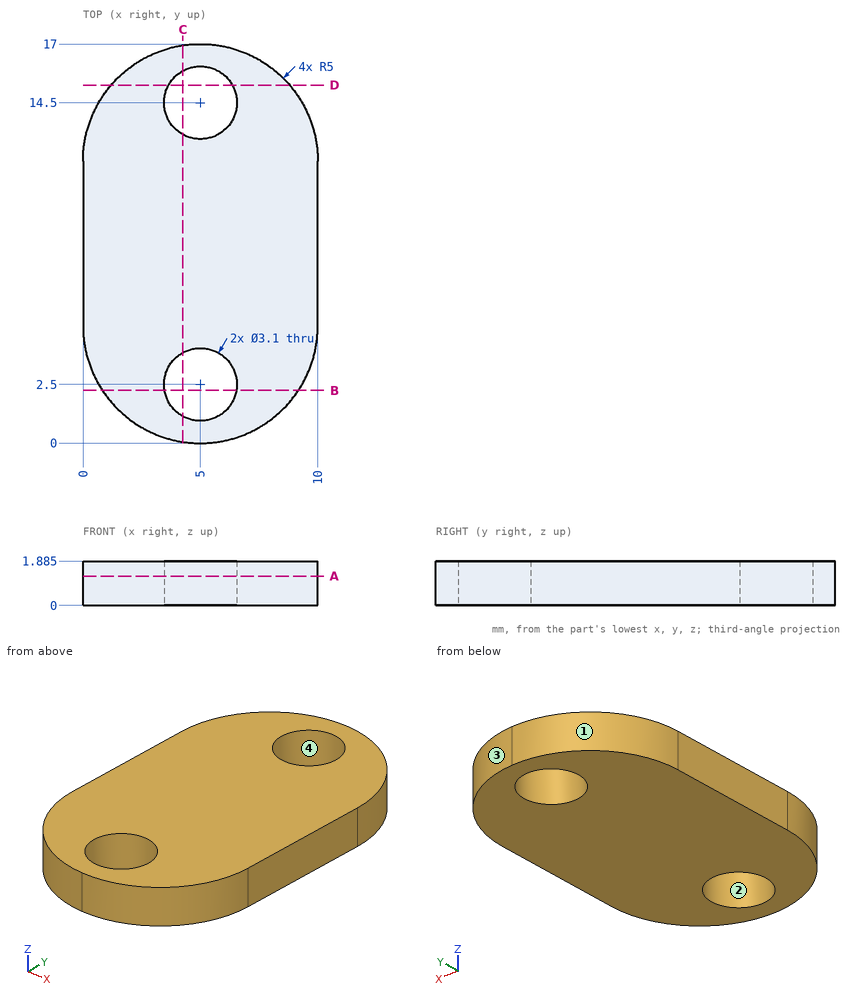
Can you work these out from the drawing? Everything is in mm from the part's minimum corner. Give positions to 0.01 mm unless a question says otherwise; leave off trailing zeros. Loops run counter-clockwise (first coordinate to the right, second up) from the corner with the lowest first, then second, coordinate; pieces in that order, holes last. Notation, with made-up numbers: (44.25, -1.5) - (76.25, -1.5) arc R32 ccw to (76.25, 32.5) - close; hole circle Ø6 at (19, 27). An arc over 180 degrees is marked (long way). Use one line per item in the form item = value.
1. I want a section at C-C (x = 4.25). Please give me the cut outline in (y, z) (1 decimal), and give its area (3 significant figures).
Response values:
outline = (0.1, 0) - (1.1, 0) - (1.1, 1.9) - (0.1, 1.9) - close; (3.9, 0) - (13.1, 0) - (13.1, 1.9) - (3.9, 1.9) - close; (15.9, 0) - (16.9, 0) - (16.9, 1.9) - (15.9, 1.9) - close
area = 21.6 mm²
2. I want a section at A-A (z = 1.25). Give the number of separate pieces and of enclosed holes in the cut face.
Response values:
separate_pieces = 1
enclosed_holes = 2
3. Thinking about a two-plate mould opening in X: for the marked faces 1, 2, 3 and 4, which applies, released by +X, released by -X, zero draft, split by the parting line, or undercut?
Response values:
face_1 = released by -X
face_2 = undercut
face_3 = released by +X
face_4 = undercut
4. I need wall thicknesses on probe 1 along Y at (x, z) = (5, 0.5); probe 2 along Y at (x, z) = (6.25, 1.25) (1 decimal); probe 3 along X at (y, z) = (14.5, 1.7). Which ranges of each line are inside material? Lowest first, please.
Response values:
probe_1 = 0 to 0.95, 4.05 to 12.95, 16.05 to 17
probe_2 = 0.2 to 1.6, 3.4 to 13.6, 15.4 to 16.8
probe_3 = 0.67 to 3.45, 6.55 to 9.33
5. I'm going to push a flat-ended pin straight in: pin 1 Ø2.5 at (x, y) = (5, 14.5) entering from -Z. Where does the tip first touch, or does it pass through?
Response values:
pin_1 = through
6. I want a section at B-B (y = 2.25). Please give me the cut outline in (x, z) (1 decimal).
Response values:
outline = (0.8, 0) - (3.5, 0) - (3.5, 1.9) - (0.8, 1.9) - close; (6.5, 0) - (9.2, 0) - (9.2, 1.9) - (6.5, 1.9) - close
7. I want a section at D-D (y = 15.25). Please give me the cut outline in (x, z) (1 decimal).
Response values:
outline = (1.2, 0) - (3.6, 0) - (3.6, 1.9) - (1.2, 1.9) - close; (6.4, 0) - (8.8, 0) - (8.8, 1.9) - (6.4, 1.9) - close
